The listing builds one solid part. Answer for the finished solid, in the listing's coordinates (mm). A direction names the side the tool comes from. Round coordinates to 2 decimals unless told otherwise and drop trailing zeros. Loops run counter-clockwise (first coordinate to the right, second up) from the corner with the lowest first, then second, coordinate; pieces in that order, holes last. Notation, with made-up numbers: (-32, 7.5) -> (-19, 7.5) arc R18 ccw to (-19, 30.5) -> close; hole circle Ø7 at (-35.5, 81). An arc over 180 degrees is marked (long way). One line per question, with ' | ' between items.
from build123d import *

# Parameters (mm, degrees)
EXTRUDE_1_DEPTH             = 21
EXTRUDE_START               = 4
SKETCH_2_R                  = 5.220451321
EXTRUDE_3_DEPTH             = 6
RIB_1_REACH                 = 57.723
SKETCH_6_WALL_W             = 126.861461592
SKETCH_6_WALL_H             = 6
FILLET_1_R                  = 6
FILLET_2_R                  = 6
HOLE_WIZARD_C_3_D           = 6.6
HOLE_WIZARD_C_3_CBORE_D     = 13
HOLE_WIZARD_C_3_CBORE_DEPTH = 0.5
FILLET_3_R                  = 6
FILLET_4_R                  = 6
MIRROR_6_COPY_1_D           = 6.6
MIRROR_6_COPY_1_CBORE_D     = 13
MIRROR_6_COPY_1_CBORE_DEPTH = 0.5
MIRROR_6_COPY_2_D           = 6.6
MIRROR_6_COPY_2_CBORE_D     = 13
MIRROR_6_COPY_2_CBORE_DEPTH = 0.5


with BuildPart() as part:
    # 草图1 → 凸台-拉伸1 (new, symmetric)
    with BuildSketch(Plane.XY):
        Polygon((-10, 2), (10, 2), (10, 0), (30, 0), (30, 8), (-30, 8), (-30, 0), (-10, 0), align=None)
    extrude(amount=EXTRUDE_1_DEPTH, both=True)

    # 草图2 → 凸台-拉伸3 (add)
    with BuildSketch(Plane(origin=(6, 0, 0), x_dir=(0, 0, -1), z_dir=(1, 0, 0)).offset(EXTRUDE_START)):
        with BuildLine():
            Line((-20, 8), (20, 8))
            Line((20, 8), (9.327204223, 35.606003519))
            ThreePointArc((9.327204223, 35.606003519), (0, 42), (-9.327204223, 35.606003519))
            Line((-9.327204223, 35.606003519), (-20, 8))
        make_face()
        with Locations((0, 32)):
            Circle(SKETCH_2_R, mode=Mode.SUBTRACT)
    extrude_3 = extrude(amount=EXTRUDE_3_DEPTH)

    # 草图6 wall → 筋1 (add, up to next)
    with BuildSketch(Plane(origin=(19, 14, 0), x_dir=(0.4472135955, -0.894427191, 0), z_dir=(0.894427191, 0.4472135955, 0)), mode=Mode.PRIVATE) as rib_1_sk1:
        Rectangle(SKETCH_6_WALL_W, SKETCH_6_WALL_H)
    rib_1_tool1 = extrude(rib_1_sk1.sketch, amount=-RIB_1_REACH, mode=Mode.PRIVATE) - part.part
    rib_1 = rib_1_tool1.solids().sort_by_distance((19, 14, 0))[0]
    add(rib_1)

    # 圆角1
    fillet_1_edges = [part.edges().sort_by_distance(p)[0] for p in [
        (30, 4, 21),
    ]]
    fillet(fillet_1_edges, radius=FILLET_1_R)

    # 圆角2
    fillet_2_edges = [part.edges().sort_by_distance(p)[0] for p in [
        (30, 4, -21),
    ]]
    fillet(fillet_2_edges, radius=FILLET_2_R)

    # 打孔尺寸(%根据六角头螺)栓 C 级的类型3 (through all)
    with Locations(Plane(origin=(0, 8, 0), x_dir=(1, 0, 0), z_dir=(0, 1, 0))):
        with Locations((23.086377714, -14.06523012)):
            hole_wizard_c_3 = CounterBoreHole(HOLE_WIZARD_C_3_D / 2, HOLE_WIZARD_C_3_CBORE_D / 2, HOLE_WIZARD_C_3_CBORE_DEPTH)

    # 镜向1: 凸台-拉伸3, 筋1, 打孔尺寸(%根据六角头螺)栓 C 级的类型3 across plane
    add(extrude_3.mirror(Plane(origin=(0, 0, 0), x_dir=(0, 0, 1), z_dir=(1, 0, 0))))
    add(rib_1.mirror(Plane(origin=(0, 0, 0), x_dir=(0, 0, 1), z_dir=(1, 0, 0))))
    add(hole_wizard_c_3.mirror(Plane(origin=(0, 0, 0), x_dir=(0, 0, 1), z_dir=(1, 0, 0))), mode=Mode.SUBTRACT)

    # 圆角3
    fillet_3_edges = [part.edges().sort_by_distance(p)[0] for p in [
        (-30, 4, 21),
    ]]
    fillet(fillet_3_edges, radius=FILLET_3_R)

    # 圆角4
    fillet_4_edges = [part.edges().sort_by_distance(p)[0] for p in [
        (-30, 4, -21),
    ]]
    fillet(fillet_4_edges, radius=FILLET_4_R)

    # 镜向2: 打孔尺寸(%根据六角头螺)栓 C 级的类型3 across plane
    add(hole_wizard_c_3.mirror(Plane.XY), mode=Mode.SUBTRACT)

    # 镜向6 copy 1 (through all)
    with Locations(Plane(origin=(0, 8, 0), x_dir=(-1, 0, 0), z_dir=(0, 1, 0))):
        with Locations((23.086377714, -14.06523012)):
            CounterBoreHole(MIRROR_6_COPY_1_D / 2, MIRROR_6_COPY_1_CBORE_D / 2, MIRROR_6_COPY_1_CBORE_DEPTH)

    # 镜向6 copy 2 (through all)
    with Locations(Plane(origin=(0, 8, 0), x_dir=(-1, 0, 0), z_dir=(0, 1, 0))):
        with Locations((23.086377714, 14.06523012)):
            CounterBoreHole(MIRROR_6_COPY_2_D / 2, MIRROR_6_COPY_2_CBORE_D / 2, MIRROR_6_COPY_2_CBORE_DEPTH)


solid = part.part
Q1. A cutting plane is placed at C-C on y = 33.5. Give the vertices of the cut face in (x, z).
Numbers:
outline: (-16, -10.14) -> (-10, -10.14) -> (-10, -5) -> (-16, -5) -> close; (-16, 5) -> (-10, 5) -> (-10, 10.14) -> (-16, 10.14) -> close; (10, -10.14) -> (16, -10.14) -> (16, -5) -> (10, -5) -> close; (10, 5) -> (16, 5) -> (16, 10.14) -> (10, 10.14) -> close
Q2. A cutting plane is placed at B-B on y = 22. Give the vertices of the cut face in (x, z), plus the area to 3 significant figures.
Numbers:
outline: (-16, -14.59) -> (-10, -14.59) -> (-10, 14.59) -> (-16, 14.59) -> close; (10, -14.59) -> (16, -14.59) -> (16, 14.59) -> (10, 14.59) -> close | area: 350 mm^2
Q3. Given pin 1 Ø6.5 at (x, z) = (21, 11.5) entering from +Y; pin 2 Ø6.5 at (x, y) = (19.5, 13) entering from -Z; pin 3 Ø1.5 at (y, z) = (15.5, -5) entering from -X, each flat-ended and moving along its own axis, determine where each tip first touches the part or whether it passes through.
Numbers:
pin 1: y = 8 | pin 2: z = -3 | pin 3: x = -16
Q4. For a pull along Z with two mould halves and no side action, classify faces 1 (the face through (-28.289, 3.944, -19.196)), 2 (the face through (26, 7.5, 17)), 3 (the face through (10, 21, 0)) as pulls with the +Z half, pulls with the -Z half, needs draft (parallel to the pull), parting line crosses it, or undercut.
Numbers:
face 1: pulls with the -Z half | face 2: undercut | face 3: needs draft
Q5. A cutting plane is placed at D-D on x = 17.5. Give the vertices of the cut face in (y, z).
Numbers:
outline: (0, -21) -> (8, -21) -> (8, -17.39) -> (7.5, -17.39) -> (7.5, -10.74) -> (8, -10.74) -> (8, -3) -> (17, -3) -> (17, 3) -> (8, 3) -> (8, 10.74) -> (7.5, 10.74) -> (7.5, 17.39) -> (8, 17.39) -> (8, 21) -> (0, 21) -> close
Q6. A cutting plane is placed at A-A on z = 0. Give the vertices of the cut face in (x, y), plus the area to 3 significant figures.
Numbers:
outline: (-30, 0) -> (-10, 0) -> (-10, 2) -> (10, 2) -> (10, 0) -> (30, 0) -> (30, 8) -> (22, 8) -> (16, 20) -> (16, 26.78) -> (10, 26.78) -> (10, 8) -> (-10, 8) -> (-10, 26.78) -> (-16, 26.78) -> (-16, 20) -> (-22, 8) -> (-30, 8) -> close; (-16, 37.22) -> (-10, 37.22) -> (-10, 42) -> (-16, 42) -> close; (10, 37.22) -> (16, 37.22) -> (16, 42) -> (10, 42) -> close | area: 795 mm^2
Q7. Find the intervals of material crossed by line 1 (X direction, y = 33, z = 6); line 2 (Y direction, x = -20, z = -18.5); line 3 (Y direction, x = -6, z = -13), in increasing order. Write a range as from..to.
Numbers:
line 1: -16..-10, 10..16 | line 2: 0..7.5 | line 3: 2..8
Q8. For faces 4 (the face through (-26, 7.5, -17)), 5 (the face through (-10, 21, 0)), 6 (the face through (0, 2, 0)), determine the directions among +Z, -Z, +X, -X, +Y, -Y from which every point of the face is accessible in a straight line to the end or side of a thin tool.
Numbers:
face 4: +Y | face 5: +Z, -Z, +Y | face 6: +Z, -Z, -Y
